from build123d import *

# Parameters (mm, degrees)
CROQUIS1_W              = 64
CROQUIS1_H              = 34
SALIENTE_EXTRUIR1_DEPTH = 3.5
CROQUIS3_W              = 5
CROQUIS3_H              = 37
SALIENTE_EXTRUIR2_DEPTH = 3.5
REDONDEO1_R             = 2
CROQUIS4_W              = 0.2
CROQUIS4_H              = 37
CORTAR_EXTRUIR1_DEPTH   = 0.5
REDONDEO2_R             = 0.1


with BuildPart() as part:
    # Croquis1 → Saliente-Extruir1 (new body)
    with BuildSketch(Plane.XY):
        Rectangle(CROQUIS1_W, CROQUIS1_H)
    extrude(amount=SALIENTE_EXTRUIR1_DEPTH)

    # Croquis3 → Saliente-Extruir2 (add)
    with BuildSketch(Plane.ZY.offset(32)):
        with Locations((2.5, 0)):
            Rectangle(CROQUIS3_W, CROQUIS3_H)
    extrude(amount=SALIENTE_EXTRUIR2_DEPTH)

    # Redondeo1
    redondeo1_edges = [part.edges().sort_by_distance(p)[0] for p in [
        (-35.5, 18.5, 2.5),
        (-35.5, -18.5, 2.5),
    ]]
    fillet(redondeo1_edges, radius=REDONDEO1_R)

    # Croquis4 → Cortar-Extruir1 (cut)
    with BuildSketch(Plane.XY.offset(5)):
        with Locations((-32.3, 0)):
            Rectangle(CROQUIS4_W, CROQUIS4_H)
        with Locations((-32.8, 0)):
            Rectangle(CROQUIS4_W, CROQUIS4_H)
        with Locations((-33.3, 0)):
            Rectangle(CROQUIS4_W, CROQUIS4_H)
        with Locations((-33.8, 0)):
            Rectangle(CROQUIS4_W, CROQUIS4_H)
        with Locations((-34.3, 0)):
            Rectangle(CROQUIS4_W, CROQUIS4_H)
        with Locations((-34.8, 0)):
            Rectangle(CROQUIS4_W, CROQUIS4_H)
        with Locations((-35.3, 0)):
            Rectangle(CROQUIS4_W, CROQUIS4_H)
    extrude(amount=-CORTAR_EXTRUIR1_DEPTH, mode=Mode.SUBTRACT)

    # Redondeo2
    redondeo2_edges = [part.edges().sort_by_distance(p)[0] for p in [
        (-32.9, 0, 5),
        (-32.7, 0, 5),
        (-33.4, 0, 5),
        (-33.2, 0, 5),
        (-33.7, 0, 5),
        (-33.9, 0, 5),
        (-34.2, 0, 5),
        (-34.4, 0, 5),
        (-34.7, 0, 5),
        (-34.9, 0, 5),
        (-35.2, 0, 5),
        (-32, 0, 5),
        (-33.45, 18.5, 5),
        (-33.45, -18.5, 5),
        (-33.60012555, 18.497492146, 5),
        (-34.051681951, 18.422406571, 5),
        (-34.554113045, 18.199660463, 5),
        (-35.061282751, 17.749958468, 5),
        (-35.061282751, -17.749958468, 5),
        (-34.554113045, -18.199660463, 5),
        (-34.051681951, -18.422406571, 5),
        (-33.60012555, -18.497492146, 5),
        (-33.05, -18.5, 5),
        (-32.55, -18.5, 5),
        (-32.1, -18.5, 5),
        (-33.05, 18.5, 5),
        (-32.55, 18.5, 5),
        (-32.1, 18.5, 5),
        (-32.4, 0, 5),
        (-32.2, 0, 5),
    ]]
    fillet(redondeo2_edges, radius=REDONDEO2_R - 0.0001)  # a hair under: the kernel refuses the full size


solid = part.part
Work out the finished part from the listing and answer in its coordinate system (mm). A direction names the side the tool comes from. Round coordinates to 2 decimals unless told otherwise and drop trailing zeros. Write each loop counter-clockwise with the first axis right and the second up, starting at its lowest first coordinate (ties: lowest second). Pieces come first, ordered by that corner, then holes. Notation, with made-up numbers: M -1,-24.5 L 44,-24.5 A33 ccw 44,7.5 Z; hole C 40,57.25 d1. An arc over 180 degrees is marked long. Use a Markdown table: item, result.
1) Flat-ended cylindrical pins translate along their axes: pin 1 (1 mm diameter, centred on x = -9, z = 1.5, fed in from +Y); pin 2 (1.8 mm diameter, centred on x = -1, z = 2.5, fed in from -Y); pin 3 (3 mm diameter, centred on x = 2, y = 13.5, fed in from +Z). Find the tip coordinate at first contact, or state that the pin passes through.
Taken from the geometry:
| item | result |
|---|---|
| pin 1 | stops at y = 17 |
| pin 2 | stops at y = -17 |
| pin 3 | stops at z = 3.5 |
2) Which of the six approach directions +Z, -Z, +X, -X, +Y, -Y give full straight-line access (tool end or side, diameter ignored) to faces 1 (the face through (0, -17, 2)), 2 (the face through (0, 0, 3.5)), 3 (the face through (-34.9, 17.93, 2.54)), 4 (the face through (0, 17, 2))?
Taken from the geometry:
| item | result |
|---|---|
| face 1 | +Z, -Z, +X, -Y |
| face 2 | +Z, +X, +Y, -Y |
| face 3 | +Z, -Z, -X, +Y |
| face 4 | +Z, -Z, +X, +Y |
3) The part is cut by section B-B on x = 10.5. Give the vertices of the cut face in (y, z), plus the area to 3 significant figures.
Taken from the geometry:
| item | result |
|---|---|
| outline | M -17,0 L 17,0 L 17,3.5 L -17,3.5 Z |
| area | 119 mm2 |
4) The part is cut by section A-A on z = 1.2. Give the vertices of the cut face in (x, y), plus the area to 3 significant figures.
Taken from the geometry:
| item | result |
|---|---|
| outline | M -35.5,-16.5 A2 ccw -33.5,-18.5 L -32,-18.5 L -32,-17 L 32,-17 L 32,17 L -32,17 L -32,18.5 L -33.5,18.5 A2 ccw -35.5,16.5 Z |
| area | 2,300 mm2 |
5) Consider line 1 (Z direction, x = -13, y = 12); line 2 (X direction, y = 10, z = 4.1); line 3 (Y direction, x = 6, z = 2.35). Determine where each line is inside the solid, lowest interval first. Write a range as [from, to].
Taken from the geometry:
| item | result |
|---|---|
| line 1 | z = [0, 3.5] |
| line 2 | x = [-35.5, -32] |
| line 3 | y = [-17, 17] |
